Work out the finished part from the listing and answer in its coordinate system (mm). Coordinates: 2 decimals unless noted, no trailing zeros. Write each loop counter-clockwise with the first axis right and the second up, starting at its lowest first coordinate (ties: lowest second). Pieces come first, ordered by that corner, then holes. Notation, with made-up numbers: (-38, -8) - (11, -8) arc R22 ccw to (11, 10) - close; hole circle Ø6 at (12.5, 36). An arc over 180 degrees is marked (long way). Use a Markdown table: item, result. Add a question column.
(1) Given pin 1 Ø5 at (y, z) = (17.25, 0) entering from +X; pin 2 Ø3 at (x, z) = (3, 4) entering from +Y, each flat-ended and moving along its own axis, determine where each tip first touches the part or whether it passes through.
(2) The part is cut by section A-A, the plane z = 0. Give the vertices of the cut face in (x, y), then the cut area to 3 significant figures.
(3) The part is cut by section D-D, the plane z = 18. Give the vertices of the cut face in (x, y), then the cut area to 3 significant figures.
(4) The part is cut by section B-B, the plane y = 17.25. Give the vertices of the cut face in (x, z), then the cut area to 3 significant figures.
(5) Find the intervals of material crossed by line 1 (Y direction, x = 3.75, z = 0); line 2 (Y direction, x = 4.5, z = 15.5); line 3 (Z direction, x = 1, y = -9), in increasing order. Write a range as from..to.
(6) The part is cut by section C-C, the plane x = 1.5. Give the vertices of the cut face in (y, z) (3 decimals).
from build123d import *

# Parameters (mm, degrees)
SKETCH_1_R          = 29.5
EXTRUDE_1_DEPTH     = 6.6
SKETCH_2_R          = 2
CUT_EXTRUDE_1_DEPTH = 21


with BuildPart() as part:
    # 草图1 → 凸台-拉伸1 (new body)
    with BuildSketch(Plane(origin=(0, 0, 0), x_dir=(0, 0, -1), z_dir=(1, 0, 0))):
        Circle(SKETCH_1_R)
    extrude(amount=EXTRUDE_1_DEPTH)

    # 草图2 → 切除-拉伸1 (cut)
    with BuildSketch(Plane(origin=(6.6, 0, 0), x_dir=(0, 0, -1), z_dir=(1, 0, 0))):
        with Locations((0, 17.25)):
            Circle(SKETCH_2_R)
        with Locations((14.938938215, 8.625)):
            Circle(SKETCH_2_R)
        with Locations((14.938938215, -8.625)):
            Circle(SKETCH_2_R)
        with Locations((0, -17.25)):
            Circle(SKETCH_2_R)
        with Locations((-14.938938215, -8.625)):
            Circle(SKETCH_2_R)
        with Locations((-14.938938215, 8.625)):
            Circle(SKETCH_2_R)
    extrude(amount=-CUT_EXTRUDE_1_DEPTH, mode=Mode.SUBTRACT)


solid = part.part
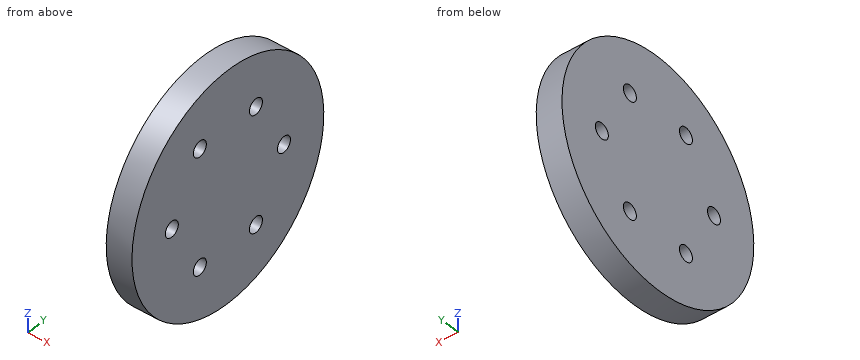
Model answer:
| question | item | result |
|---|---|---|
| 1 | pin 1 | x = 6.6 |
| 1 | pin 2 | y = 29.39 |
| 2 | outline | (0, -29.5) - (6.6, -29.5) - (6.6, -19.25) - (0, -19.25) - close; (0, -15.25) - (6.6, -15.25) - (6.6, 15.25) - (0, 15.25) - close; (0, 19.25) - (6.6, 19.25) - (6.6, 29.5) - (0, 29.5) - close |
| 2 | area | 337 mm^2 |
| 3 | outline | (0, -23.37) - (6.6, -23.37) - (6.6, 23.37) - (0, 23.37) - close |
| 3 | area | 309 mm^2 |
| 4 | outline | (0, -23.93) - (6.6, -23.93) - (6.6, -2) - (0, -2) - close; (0, 2) - (6.6, 2) - (6.6, 23.93) - (0, 23.93) - close |
| 4 | area | 289 mm^2 |
| 5 | line 1 | -29.5..-19.25, -15.25..15.25, 19.25..29.5 |
| 5 | line 2 | -25.1..-10.54, -6.71..6.71, 10.54..25.1 |
| 5 | line 3 | -28.09..-16.9, -12.97..12.97, 16.9..28.09 |
| 6 | outline | circle Ø59 at (0, 0); hole circle Ø4 at (-17.25, 0); hole circle Ø4 at (-8.625, -14.939); hole circle Ø4 at (-8.625, 14.939); hole circle Ø4 at (8.625, -14.939); hole circle Ø4 at (8.625, 14.939); hole circle Ø4 at (17.25, 0) |
